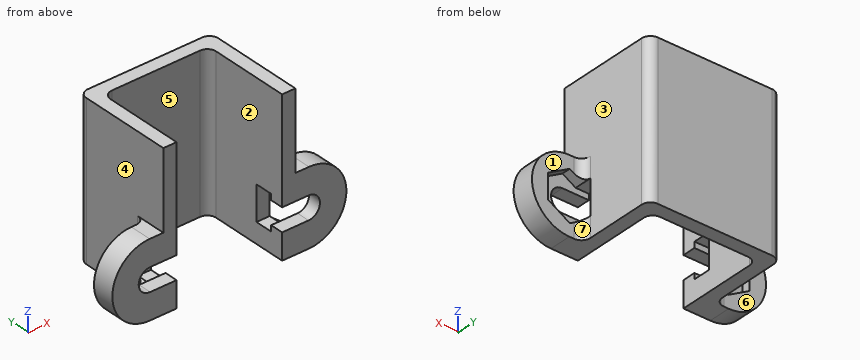
```python
from build123d import *

# Parameters (mm, degrees)
BOSS_EXTRUDE1_DEPTH     = 17.3
BOSS_EXTRUDE2_DEPTH     = 2.5
CUT_EXTRUDE1_DEPTH      = 2.5
CUT_EXTRUDE2_DEPTH      = 1
CUT_EXTRUDE2_DEPTH_BACK = 1
FILLET1_R               = 1
FILLET2_R               = 1


with BuildPart() as part:
    # Sketch1 → Boss-Extrude1 (new body)
    with BuildSketch(Plane.XY):
        Polygon((6, 0), (7.5, 0), (7.5, 11.5), (-7.5, 11.5), (-7.5, 0), (-6, 0), (-6, 10), (6, 10), align=None)
    extrude(amount=BOSS_EXTRUDE1_DEPTH)

    # Sketch2 → Boss-Extrude2 (add)
    with BuildSketch(Plane.XZ):
        with BuildLine():
            Line((-7.5, 0), (-9.05, 0))
            ThreePointArc((-9.05, 0), (-13.3, 4.25), (-9.05, 8.5))
            Line((-9.05, 8.5), (-7.5, 8.5))
            Line((-7.5, 8.5), (-7.5, 0))
        make_face()
        with BuildLine():
            Line((7.5, 0), (9.05, 0))
            ThreePointArc((9.05, 0), (13.3, 4.25), (9.05, 8.5))
            Line((9.05, 8.5), (7.5, 8.5))
            Line((7.5, 8.5), (7.5, 0))
        make_face()
    extrude(amount=-BOSS_EXTRUDE2_DEPTH)

    # Sketch3 → Cut-Extrude1 (cut)
    with BuildSketch(Plane(origin=(0, 2.5, 0), x_dir=(1, 0, 0), z_dir=(0, 1, 0))):
        with BuildLine():
            Line((6, -2.95), (9, -2.95))
            ThreePointArc((9, -2.95), (10.3, -4.25), (9, -5.55))
            Line((9, -5.55), (6, -5.55))
            Line((6, -5.55), (6, -2.95))
        make_face()
        with BuildLine():
            Line((-6, -2.95), (-9, -2.95))
            ThreePointArc((-9, -2.95), (-10.3, -4.25), (-9, -5.55))
            Line((-9, -5.55), (-6, -5.55))
            Line((-6, -5.55), (-6, -2.95))
        make_face()
    extrude(amount=-CUT_EXTRUDE1_DEPTH, mode=Mode.SUBTRACT)

    # Sketch4 → Cut-Extrude2 (cut, two sides: drawn at the far end of the back side and taken through both)
    with BuildSketch(Plane(origin=(0, 2.5, 0), x_dir=(1, 0, 0), z_dir=(0, 1, 0)).offset(-CUT_EXTRUDE2_DEPTH_BACK)):
        Polygon((9, -1.420983681), (7.5, -2.287009085), (6, -2.287009085), (6, -6.212990915), (7.5, -6.212990915), (9, -7.079016319), (11.45, -5.66450816), (11.45, -2.83549184), align=None)
        Polygon((-6, -6.212990915), (-7.5, -6.212990915), (-9, -7.079016319), (-11.45, -5.66450816), (-11.45, -2.83549184), (-9, -1.420983681), (-7.5, -2.287009085), (-6, -2.287009085), align=None)
    extrude(amount=CUT_EXTRUDE2_DEPTH + CUT_EXTRUDE2_DEPTH_BACK, mode=Mode.SUBTRACT)

    # Fillet1
    fillet1_edges = [part.edges().sort_by_distance(p)[0] for p in [
        (6, 10, 8.65),
        (-6, 10, 8.65),
        (-7.5, 2.5, 1.143504542),
        (7.5, 2.5, 7.356495458),
        (7.5, 2.5, 1.143504542),
        (-7.5, 2.5, 7.356495458),
    ]]
    fillet(fillet1_edges, radius=FILLET1_R - 0.0001)  # a hair under: the kernel refuses the full size

    # Fillet2
    fillet2_edges = [part.edges().sort_by_distance(p)[0] for p in [
        (-7.5, 11.5, 8.65),
        (7.5, 11.5, 8.65),
    ]]
    fillet(fillet2_edges, radius=FILLET2_R)


solid = part.part
```
Input: part model. Units: mm. Frame: model coordinates. Face numbers are marked on the shaded views. A direction names the side the tool comes from. Give positions to 0.01 mm unless a question says otherwise; leave off trailing zeros. Order: outer loops, then holes, each group sorted by start corner. A loop starts at its lowest first (then second) coordinate and runs counter-clockwise, first axis right, second up. Notation, with made-up numbers: (-39.5, 4) - (-23.5, 4) arc R21 cw to (-23.5, 22) - close; hole circle Ø7 at (86, -19.5). An arc over 180 degrees is marked (long way). Use a Markdown table: item, result.
(1) Section query C-C (x = -10). Output: boundary loops of the cut face in (y, z), then the cut area to 3 significant figures.
Computed values:
| item | result |
|---|---|
| outline | (0, 0.11) - (2.5, 0.11) - (2.5, 2) - (1.5, 2) - (1.5, 3.42) - (0, 3.42) - close; (0, 5.08) - (1.5, 5.08) - (1.5, 6.5) - (2.5, 6.5) - (2.5, 8.39) - (0, 8.39) - close |
| area | 13.7 mm2 |
(2) Draft query along X for the marked faces 5, 6 and 7. Return one class per face: released by +X, released by -X, zero draft, split by the parting line, or undercut.
Computed values:
| item | result |
|---|---|
| face 5 | undercut |
| face 6 | zero draft |
| face 7 | released by +X |
(3) Section query B-B (z = 4.5). Output: boundary loops of the cut face in (x, y).
Computed values:
| item | result |
|---|---|
| outline | (-13.29, 0) - (-10.28, 0) - (-10.28, 1.5) - (-11.45, 1.5) - (-11.45, 2.5) - (-13.29, 2.5) - close; (-7.5, 3.5) - (-6, 3.5) - (-6, 9) arc R1 cw to (-5, 10) - (5, 10) arc R1 cw to (6, 9) - (6, 3.5) - (7.5, 3.5) - (7.5, 10.5) arc R1 ccw to (6.5, 11.5) - (-6.5, 11.5) arc R1 ccw to (-7.5, 10.5) - close; (10.28, 0) - (13.29, 0) - (13.29, 2.5) - (11.45, 2.5) - (11.45, 1.5) - (10.28, 1.5) - close |
(4) Section query A-A (y = 4.75). Output: boundary loops of the cut face in (x, z).
Computed values:
| item | result |
|---|---|
| outline | (-7.5, 0) - (-6, 0) - (-6, 17.3) - (-7.5, 17.3) - close; (6, 0) - (7.5, 0) - (7.5, 17.3) - (6, 17.3) - close |
(5) Pin query (flat end, axial travel): pin 1 (1.2 mm diameter, centred on x = -7, z = 4, fed in from -Y); pin 2 (1.5 mm diameter, centred on x = -1.5, z = 14, fed in from -Y); pin 3 (2 mm diameter, centred on y = 4.5, z = 3, fed in from +X). Return the tip coordinate at first contact, or that it passes through.
Computed values:
| item | result |
|---|---|
| pin 1 | stops at y = 3.5 |
| pin 2 | stops at y = 10 |
| pin 3 | stops at x = 7.5 |
(6) Access query for the marked faces 1, 2, 3 and 4. Directions: +Z, -Z, +X, -X, +Y, -Y. A direction counts if a zero-diameter tool reaches every point of the face in a straight line with its end or side. Return the directions, or none.
Computed values:
| item | result |
|---|---|
| face 1 | +Z, -Z, +X, +Y |
| face 2 | +Z, -Z, -Y |
| face 3 | +Z, +X, +Y |
| face 4 | +Z, -X, +Y |
(7) Section query D-D (x = 0). Output: boundary loops of the cut face in (y, z), then the cut area to 4 significant figures.
Computed values:
| item | result |
|---|---|
| outline | (10, 0) - (11.5, 0) - (11.5, 17.3) - (10, 17.3) - close |
| area | 25.95 mm2 |
(8) Line query: line 1 (X direction, y = 4.25, z = 10.5); line 2 (Z direction, x = -6.5, y = 3); line 3 (Z direction, x = -8.5, y = 0.5). Output: solid intervals per line, ascending. Write a range as from..to.
Computed values:
| item | result |
|---|---|
| line 1 | x = -7.5..-6, 6..7.5 |
| line 2 | z = 0..2.29, 6.21..17.3 |
| line 3 | z = 0..2.95, 5.55..8.5 |
